Geometry check sheet. Reference: the model listing, model coordinates, mm. Face numbers are marked on the shaded views. A direction names the side the tool comes from. Round coordinates to 2 decimals unless told otherwise and drop trailing zeros. Write each loop counter-clockwise with the first axis right and the second up, starting at its lowest first coordinate (ties: lowest second). Pieces come first, ordered by that corner, then holes. Notation, with made-up numbers: M 51,71 L 87,71 A16 cw 87,86 Z; hole C 57.25,-40 d9. An arc over 180 degrees is marked long. One line per item, written item: value. Start each with the question number.
1. Scan lines: probe 1 along Y at (x, z) = (1, 16.5); probe 2 along Y at (x, z) = (39, 12.5) (3 decimals); probe 3 along Z at (x, y) = (27, 4). Record each from-to range of solid material in increasing order. Write a range as [from, to].
2. Section check C-C (x = 28.5). Record the boundary of the cut face in (y, z), and give its area (3 significant figures).
3. Section check B-B (z = 7.75). Record the boundary of the cut face in (x, y) (3 decimals).
4. Access from +Z, -Z, +X, -X, +Y, -Y to the whole of each face (thin tool, end or side, straight path). Record for the marked faces 1, 2 and 3.
5. Release check for a two-part mould opening along X. For the marked faces 4, 5, 6 and 7 record: pulls with the +X half, pulls with the -X half, needs draft (parallel to the pull), parting line crosses it, or undercut.
6. Section check A-A (y = -11). Record the boundary of the cut face in (x, z) (1 decimal).
7. Depth check by flat-ended pin: P1, Ø2, axis at y = -11, z = 11.5, coming from the -X side; P2, Ø2.5, axis at x = 13.84, z = 2.48, coming from the +Y side; P3, Ø3, axis at x = 23.5, y = 8.5, coming from the +Z side; P4, Ø8, axis at x = 2.5, y = 9, coming from the -Z side. Enter the tip coordinate at first touch or a pass-through.
8. Section check D-D (y = 6). Count the separate pieces of the cut face and the enclosed holes in it, and give its area (3 significant figures).
from build123d import *

# Parameters (mm, degrees)
F0_W      = 36.83
F0_H      = 17.018
F1_DEPTH  = 22.479
F2_R      = 7.112
F1_FACE_W = 17.018
F1_FACE_H = 8.255
F4_DEPTH  = 27.432
F6_DEPTH  = 16.002
F7_R      = 12.816169
F7_R_2    = 4.7625
F8_DEPTH  = 1.524
F9_R      = 1.524
F10_R     = 1.016
F11_DEPTH = 2.032
F12_W     = 2.54
F12_H     = 5.08
F13_DEPTH = 2.54
F15_DEPTH = 1.143
F16_W     = 2.54
F16_H     = 5.08
F17_DEPTH = 2.54
F19_DEPTH = 8.89
F21_DEPTH = 8.89
F22_R     = 1.324614
F23_DEPTH = 1.9558
F24_R     = 1.419753
F25_DEPTH = 25.4


with BuildPart() as f1:
    # F0 (on Top) → F1 (new body)
    with BuildSketch(Plane.XY):
        with Locations((0, -0.762)):
            Rectangle(F0_W, F0_H)
    extrude(amount=F1_DEPTH)

    # F2
    f2_edges = [f1.edges().sort_by_distance(p)[0] for p in [
        (-18.415, -0.762, 22.479),
        (-18.415, -0.762, 0),
    ]]
    fillet(f2_edges, radius=F2_R)

    # F3 (on face) + F1_face (on face) → F4 (join)
    with BuildSketch(Plane.YZ.offset(18.415)):
        with BuildLine():
            Line((-9.271, 18.582747), (-9.271, 3.896253))
            ThreePointArc((-9.271, 3.896253), (-5.441313, 1.020381), (-0.762, 0))
            ThreePointArc((-0.762, 0), (3.917313, 1.020381), (7.747, 3.896253))
            Line((7.747, 3.896253), (7.747, 18.582747))
            ThreePointArc((7.747, 18.582747), (3.917313, 21.458619), (-0.762, 22.479))
            ThreePointArc((-0.762, 22.479), (-5.441313, 21.458619), (-9.271, 18.582747))
        make_face()
    with BuildSketch(Plane(origin=(18.415, -0.762, 11.2395), x_dir=(0, 1, 0), z_dir=(1, 0, 0))):
        Rectangle(F1_FACE_W, F1_FACE_H)
    extrude(amount=F4_DEPTH)

    # F5 (on face) → F6 (cut)
    with BuildSketch(Plane.YZ.offset(45.847)):
        with BuildLine():
            ThreePointArc((13.335, 20.428588), (-0.762, 28.067), (-14.859, 20.428588))
            Line((-14.859, 20.428588), (-14.859, 2.050412))
            ThreePointArc((-14.859, 2.050412), (-0.762, -5.588), (13.335, 2.050412))
            Line((13.335, 2.050412), (13.335, 20.428588))
        make_face()
        with BuildLine():
            ThreePointArc((-9.271, 18.582747), (-0.762, 22.479), (7.747, 18.582747))
            Line((7.747, 18.582747), (7.747, 3.896253))
            ThreePointArc((7.747, 3.896253), (-0.762, 0), (-9.271, 3.896253))
            Line((-9.271, 3.896253), (-9.271, 18.582747))
        make_face(mode=Mode.SUBTRACT)
        with BuildLine():
            Line((7.747, 3.896253), (7.747, 18.582747))
            ThreePointArc((7.747, 18.582747), (-0.762, 22.479), (-9.271, 18.582747))
            Line((-9.271, 18.582747), (-9.271, 3.896253))
            ThreePointArc((-9.271, 3.896253), (-0.762, 0), (7.747, 3.896253))
        make_face()
        with BuildLine():
            Line((-8.509, 4.185282), (-8.509, 18.293718))
            ThreePointArc((-8.509, 18.293718), (-0.762, 21.717), (6.985, 18.293718))
            Line((6.985, 18.293718), (6.985, 4.185282))
            ThreePointArc((6.985, 4.185282), (-0.762, 0.762), (-8.509, 4.185282))
        make_face(mode=Mode.SUBTRACT)
    extrude(amount=-F6_DEPTH, mode=Mode.SUBTRACT)

    # F7 (on face) → F8 (cut)
    with BuildSketch(Plane.YZ.offset(45.847)):
        with Locations((-0.762, 11.2395)):
            Circle(F7_R)
        with BuildLine():
            ThreePointArc((6.985, 4.185282), (-0.762, 0.762), (-8.509, 4.185282))
            Line((-8.509, 4.185282), (-8.509, 18.293718))
            ThreePointArc((-8.509, 18.293718), (-0.762, 21.717), (6.985, 18.293718))
            Line((6.985, 18.293718), (6.985, 4.185282))
        make_face(mode=Mode.SUBTRACT)
        with BuildLine():
            Line((-8.509, 18.293718), (-8.509, 4.185282))
            ThreePointArc((-8.509, 4.185282), (-0.762, 0.762), (6.985, 4.185282))
            Line((6.985, 4.185282), (6.985, 18.293718))
            ThreePointArc((6.985, 18.293718), (-0.762, 21.717), (-8.509, 18.293718))
        make_face()
        with Locations((-0.762, 11.2395)):
            Circle(F7_R_2, mode=Mode.SUBTRACT)
    extrude(amount=-F8_DEPTH, mode=Mode.SUBTRACT)

    # F9
    f9_edges = [f1.edges().sort_by_distance(p)[0] for p in [
        (44.323, -0.762, 0.762),
    ]]
    fillet(f9_edges, radius=F9_R)

    # F10 (on face) → F11 (join)
    with BuildSketch(Plane.YZ.offset(45.847)):
        with Locations((-0.762, 11.2395)):
            Circle(F10_R)
    extrude(amount=F11_DEPTH)

    # F12 (on face) → F13 (join)
    with BuildSketch(Plane.XZ.offset(9.271)):
        with Locations((23.495, 11.2395)):
            Rectangle(F12_W, F12_H)
    extrude(amount=F13_DEPTH)

    # F14 (on face) → F15 (join)
    with BuildSketch(Plane(origin=(0, 7.747, 0), x_dir=(-1, 0, 0), z_dir=(0, 1, 0))):
        with BuildLine():
            Line((-18.415, 0), (11.303, 0))
            ThreePointArc((11.303, 0), (16.331943, 2.083057), (18.415, 7.112))
            Line((18.415, 7.112), (18.415, 15.367))
            ThreePointArc((18.415, 15.367), (16.331943, 20.395943), (11.303, 22.479))
            Line((11.303, 22.479), (-18.415, 22.479))
            Line((-18.415, 22.479), (-18.415, 18.582747))
            Line((-18.415, 18.582747), (-18.415, 3.896253))
            Line((-18.415, 3.896253), (-18.415, 0))
        make_face()
    extrude(amount=F15_DEPTH)

    # F16 (on face) → F17 (join)
    with BuildSketch(Plane(origin=(0, 7.747, 0), x_dir=(-1, 0, 0), z_dir=(0, 1, 0))):
        with Locations((-23.495, 11.2395)):
            Rectangle(F16_W, F16_H)
    extrude(amount=F17_DEPTH)

    # F18 (on face) → F19 (join)
    with BuildSketch(Plane.XZ.offset(9.271)):
        with BuildLine():
            Line((-5.4102, 9.280857), (-5.4102, 13.198143))
            ThreePointArc((-5.4102, 13.198143), (-7.239, 13.9192), (-9.0678, 13.198143))
            Line((-9.0678, 13.198143), (-9.0678, 9.280857))
            ThreePointArc((-9.0678, 9.280857), (-7.239, 8.5598), (-5.4102, 9.280857))
        make_face()
    extrude(amount=F19_DEPTH)

    # F20 (on face) → F21 (join)
    with BuildSketch(Plane(origin=(0, 8.89, 0), x_dir=(-1, 0, 0), z_dir=(0, 1, 0))):
        with BuildLine():
            Line((5.4102, 13.198143), (5.4102, 9.280857))
            ThreePointArc((5.4102, 9.280857), (7.239, 8.5598), (9.0678, 9.280857))
            Line((9.0678, 9.280857), (9.0678, 13.198143))
            ThreePointArc((9.0678, 13.198143), (7.239, 13.9192), (5.4102, 13.198143))
        make_face()
    extrude(amount=F21_DEPTH)

    # F22 (on face) → F23 (join)
    with BuildSketch(Plane(origin=(0, 8.89, 0), x_dir=(-1, 0, 0), z_dir=(0, 1, 0))):
        with Locations((-4.0386, 11.2395)):
            Circle(F22_R)
    extrude(amount=F23_DEPTH)

    # F24 (on face) → F25 (cut)
    with BuildSketch(Plane.XZ.offset(9.271)):
        with Locations((13.843, 20.0025)):
            Circle(F24_R)
        with Locations((13.843, 2.4765)):
            Circle(F24_R)
    extrude(amount=-F25_DEPTH, mode=Mode.SUBTRACT)


solid = f1.part
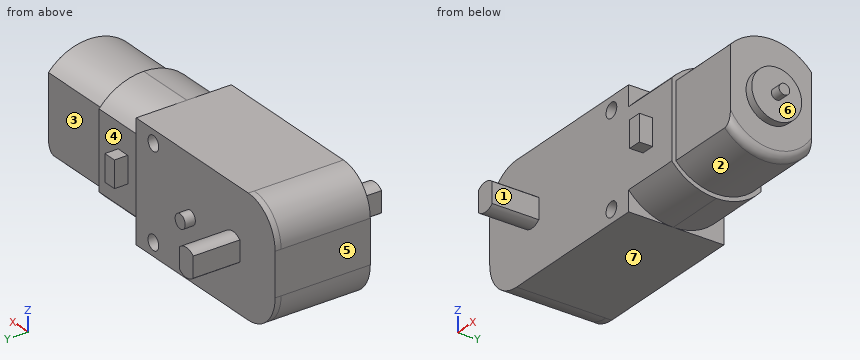
Result sheet:
1. probe 1: y = [-9.27, 8.89]
1. probe 2: y = [-8.509, 6.985]
1. probe 3: z = [1.06, 21.42]
2. outline: M -9.27,3.9 A11.24 ccw -0.76,0 A11.24 ccw 7.75,3.9 L 7.75,18.58 A11.24 ccw -0.76,22.48 A11.24 ccw -9.27,18.58 Z
2. area: 342 mm2
3. outline: M -18.415,-9.271 L 29.845,-9.271 L 29.845,-8.509 L 44.323,-8.509 L 44.323,-4.003 L 45.847,-4.003 L 45.847,2.479 L 44.323,2.479 L 44.323,6.985 L 29.845,6.985 L 29.845,7.747 L 18.415,7.747 L 18.415,8.89 L -18.415,8.89 Z
4. face 1: +Z, -Z, -Y
4. face 2: -Z, +X
4. face 3: +Z, -Z, +X, +Y
5. face 4: undercut
5. face 5: pulls with the -X half
5. face 6: pulls with the +X half
5. face 7: needs draft
6. outline: M -9.1,9.3 A2.7 ccw -5.4,9.3 L -5.4,13.2 A2.7 ccw -9.1,13.2 Z; M 22.2,8.7 L 24.8,8.7 L 24.8,13.8 L 22.2,13.8 Z
7. P1: stops at x = -9.07
7. P2: passes through
7. P3: stops at z = 19.37
7. P4: stops at z = 0
8. separate pieces: 1
8. enclosed holes: 2
8. area: 1,230 mm2
